from build123d import *

# Parameters (mm, degrees)
SKETCH1_R               = 15
BOSS_EXTRUDE1_DEPTH     = 8
SKETCH1_5_R             = 15
SKETCH1_5_R_2           = 1.6
BOSS_EXTRUDE4_DEPTH     = 4
CHAMFER1_SIZE           = 0.75
CHAMFER3_SIZE           = 1
CUT_EXTRUDE1_DEPTH      = 109.32973067
CUT_EXTRUDE1_DEPTH_BACK = 109.32973067
SKETCH8_R               = 4
CUT_EXTRUDE2_DEPTH      = 109.32973067
CUT_EXTRUDE2_DEPTH_BACK = 109.32973067
SKETCH10_R              = 1.6
CHAMFER4_SIZE           = 1.5
CHAMFER5_SIZE           = 1
CHAMFER6_SIZE           = 1


with BuildPart() as part:
    # Sketch1 → Boss-Extrude1 (new body)
    with BuildSketch(Plane.XY):
        with BuildLine():
            Line((-84.149061225, 12.330202688), (-3.782129278, -15.349324934))
            ThreePointArc((-3.782129278, -15.349324934), (19.733864864, -3.882066346), (8.266606276, 19.633927796))
            Line((8.266606276, 19.633927796), (-72.100325672, 47.313455418))
            ThreePointArc((-72.100325672, 47.313455418), (-95.616319813, 35.84619683), (-84.149061225, 12.330202688))
        make_face()
        with Locations((2.242238499, 2.142301431)):
            Circle(SKETCH1_R, mode=Mode.SUBTRACT)
        with Locations((-78.124693448, 29.821829053)):
            Circle(SKETCH1_R, mode=Mode.SUBTRACT)
    extrude(amount=BOSS_EXTRUDE1_DEPTH)

    # Sketch1_5 → Boss-Extrude4 (add)
    # profile 1 of 2: a face of its own
    with BuildSketch(Plane.XY):
        with Locations((2.242238499, 2.142301431)):
            Circle(SKETCH1_5_R)
        with Locations((2.242238499, 10.142301431)):
            Circle(SKETCH1_5_R_2, mode=Mode.SUBTRACT)
        with Locations((-5.757761501, 2.142301431)):
            Circle(SKETCH1_5_R_2, mode=Mode.SUBTRACT)
        with Locations((10.242238499, 2.142301431)):
            Circle(SKETCH1_5_R_2, mode=Mode.SUBTRACT)
        with Locations((2.242238499, -5.857698569)):
            Circle(SKETCH1_5_R_2, mode=Mode.SUBTRACT)
    # profile 2 of 2: a face of its own
    with BuildSketch(Plane.XY):
        with Locations((-78.124693448, 29.821829053)):
            Circle(SKETCH1_5_R)
    extrude(amount=BOSS_EXTRUDE4_DEPTH)

    # Chamfer1
    chamfer1_edges = [part.edges().sort_by_distance(p)[0] for p in [
        (0.642238499, -5.857698569, 4),
        (8.642238499, 2.142301431, 4),
        (-7.357761501, 2.142301431, 4),
        (0.642238499, 10.142301431, 4),
    ]]
    chamfer(chamfer1_edges, length=CHAMFER1_SIZE)

    # Chamfer3
    chamfer3_edges = [part.edges().sort_by_distance(p)[0] for p in [
        (-12.757761501, 2.142301431, 8),
        (-93.124693448, 29.821829053, 8),
    ]]
    chamfer(chamfer3_edges, length=CHAMFER3_SIZE)

    # Sketch8 → Cut-Extrude1 (cut, two sides: drawn at the far end of the back side and taken through both)
    with BuildSketch(Plane(origin=(0, 0, 0), x_dir=(-1, 0, 0), z_dir=(0, 0, -1)).offset(-CUT_EXTRUDE1_DEPTH_BACK)):
        with Locations(Location((-2.242238499, 2.142301431, 0), (0, 0, 180))):
            Circle(SKETCH8_R)
    extrude(amount=CUT_EXTRUDE1_DEPTH + CUT_EXTRUDE1_DEPTH_BACK, mode=Mode.SUBTRACT)

    # Sketch10 → Cut-Extrude2 (cut, two sides: drawn at the far end of the back side and taken through both)
    with BuildSketch(Plane(origin=(0, 0, 0), x_dir=(-1, 0, 0), z_dir=(0, 0, -1)).offset(-CUT_EXTRUDE2_DEPTH_BACK)):
        with Locations((36.683056878, 27.182871474)):
            Circle(SKETCH10_R)
        with Locations(Location((74.502789559, 40.208531531, 0), (0, 0, 180))):
            Circle(SKETCH10_R)
        with Locations(Location((81.66690259, 19.407678557, 0), (0, 0, 180))):
            Circle(SKETCH10_R)
        with Locations((43.847169909, 6.382018499)):
            Circle(SKETCH10_R)
    extrude(amount=CUT_EXTRUDE2_DEPTH + CUT_EXTRUDE2_DEPTH_BACK, mode=Mode.SUBTRACT)

    # Chamfer4
    chamfer4_edges = [part.edges().sort_by_distance(p)[0] for p in [
        (-35.083056878, 27.182871474, 8),
        (-76.102789559, 40.208531531, 4),
        (-83.26690259, 19.407678557, 4),
        (-42.247169909, 6.382018499, 8),
    ]]
    chamfer(chamfer4_edges, length=CHAMFER4_SIZE)

    # Chamfer5
    chamfer5_edges = [part.edges().sort_by_distance(p)[0] for p in [
        (-95.616319813, 35.84619683, 0),
        (-31.916859698, 33.473691607, 0),
        (19.733864864, -3.882066346, 0),
        (-43.965595251, -1.509561123, 0),
    ]]
    chamfer(chamfer5_edges, length=CHAMFER5_SIZE)

    # Chamfer6
    chamfer6_edges = [part.edges().sort_by_distance(p)[0] for p in [
        (-43.965595251, -1.509561123, 8),
        (19.733864864, -3.882066346, 8),
        (-31.916859698, 33.473691607, 8),
        (-95.616319813, 35.84619683, 8),
    ]]
    chamfer(chamfer6_edges, length=CHAMFER6_SIZE)


solid = part.part
Read the model definition and answer for the solid it produces. Units are mm, in the model's axes. A direction names the side the tool comes from. Round coordinates to 2 decimals unless told otherwise and drop trailing zeros.
1) For faces 1 (the face through (-31.5, 32.8, 7.5)), 2 (the face through (10.31, 14.79, 5.48)), determine the directions among +Z, -Z, +X, -X, +Y, -Y from which every point of the face is accessible in a straight line to the end or side of a thin tool.
2) Straight lines are drawn through the part: L1, parallel to Z at x = -5, y = 7; L2, parallel to Y at x = 4.5, z = 3.5; L3, parallel to Y at x = -78.5, z = 5.75. For each, find the intervals that lie inside material, in ascending order.
3) Flat-ended cylindrical pins translate along their axes: pin 1 (1.5 mm diameter, centred on y = 13.5, z = 1.5, fed in from -X); pin 2 (3.5 mm diameter, centred on x = -74.5, y = 40.21, fed in from +Z); pin 3 (1 mm diameter, centred on x = -44.5, y = -1, fed in from +Z). Find the tip coordinate at first contact, or state that the pin passes through.
Resolved:
1. face 1: +Z, +X, +Y
1. face 2: +Z
2. L1: z = 0 to 4
2. L2: y = -16.22 to -1.16, 5.44 to 20.93
2. L3: y = 10.38 to 14.83, 44.82 to 48.32
3. pin 1: stops at x = -88.11
3. pin 2: stops at z = 2.65
3. pin 3: stops at z = 7.81
